```python
from build123d import *

# Parameters (mm, degrees)
SKETCH1_R           = 1
BOSS_EXTRUDE1_DEPTH = 3
FILLET_2_R          = 70


with BuildPart() as part:
    # Sketch1 → Boss-Extrude1 (new body)
    with BuildSketch(Plane.XY):
        with BuildLine():
            Line((-59.269719731, 24.533720681), (-59.269719731, 18.533720681))
            Line((-59.269719731, 18.533720681), (-45.247809755, 18.533720681))
            Line((-45.247809755, 18.533720681), (-45.247809755, -4.966279319))
            Line((-45.247809755, -4.966279319), (-59.247809755, -4.966279319))
            Line((-59.247809755, -4.966279319), (-59.247809755, -9.307077777))
            Line((-59.247809755, -9.307077777), (-51.83788451, -34.085396001))
            Line((-51.83788451, -34.085396001), (-51.83788451, -65.202303041))
            ThreePointArc((-51.83788451, -65.202303041), (-50.943230184, -66.196738704), (-49.860079932, -65.411822033))
            Line((-49.860079932, -65.411822033), (-37.838240661, -9.307077777))
            Line((-37.838240661, -9.307077777), (-37.838240661, 24.533720681))
            ThreePointArc((-37.838240661, 24.533720681), (-48.553980196, 35.249460216), (-59.269719731, 24.533720681))
        make_face()
        with Locations((-52.247809755, 20.533720681)):
            Circle(SKETCH1_R, mode=Mode.SUBTRACT)
        with Locations((-52.247809755, -6.966279319)):
            Circle(SKETCH1_R, mode=Mode.SUBTRACT)
        with BuildLine():
            Line((-45.247809755, 24.533720681), (-56.258764743, 24.533720681))
            ThreePointArc((-56.258764743, 24.533720681), (-50.753287249, 30.039198175), (-45.247809755, 24.533720681))
        make_face(mode=Mode.SUBTRACT)
    extrude(amount=BOSS_EXTRUDE1_DEPTH)

    # Скругление2
    # the kernel refuses this fillet: 70 mm, written as the material it adds along each edge
    with BuildSketch(Plane(origin=(-51.83788451, -34.085396001, 0), x_dir=(-0.28651166180092774, 0.9580767545724459, 0), z_dir=(0, 0, 1))) as fillet_2_piece_1:
        with BuildLine():
            CenterArc((FILLET_2_R * 0.146322998387, FILLET_2_R), FILLET_2_R, 253.350770917, 16.649229083)
            Line((-FILLET_2_R * 0.140188663414, FILLET_2_R * 0.0419232454276), (0, 0))
            Line((0, 0), (FILLET_2_R * 0.146322998387, 0))
        make_face()
    extrude(amount=3)
    # the kernel refuses this fillet: 70 mm, written as the material it takes off along each edge
    with BuildSketch(Plane(origin=(-59.247809755, -9.307077777, -22.444406255), x_dir=(0, 1, 0), z_dir=(0, 0, 1))) as fillet_2_2_piece_1:
        with BuildLine():
            CenterArc((11.454430765, -69.637606474), FILLET_2_R, 95.832656056, 10.816573027)
            Line((-8.601385561, -2.572233654), (0, 0))
            Line((0, 0), (4.340798458, 0))
        make_face()
    extrude(amount=47.88881251, mode=Mode.SUBTRACT)
    with BuildSketch(Plane(origin=(-37.838240661, -9.307077777, -18.538648377), x_dir=(0, 1, 0), z_dir=(0, 0, 1))) as fillet_2_2_piece_2:
        with BuildLine():
            CenterArc((FILLET_2_R * 0.10593513358, FILLET_2_R), FILLET_2_R, 257.905834548, 12.094165452)
            Line((-FILLET_2_R * 0.103583858541, FILLET_2_R * 0.0221954224179), (0, 0))
            Line((0, 0), (FILLET_2_R * 0.10593513358, 0))
        make_face()
    extrude(amount=40.077296753, mode=Mode.SUBTRACT)


solid = part.part
```
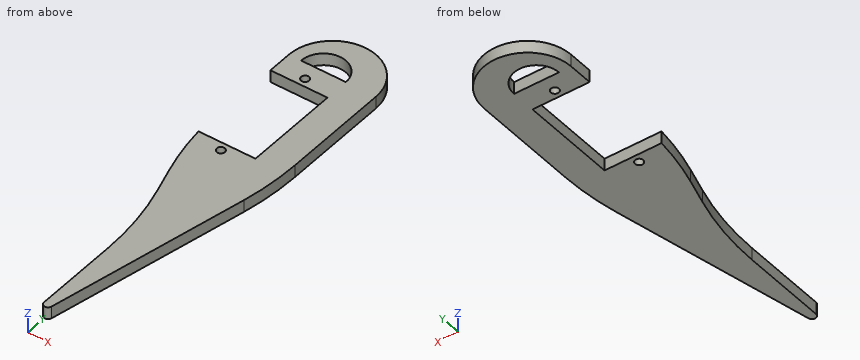
The listing builds one solid part. Answer for the finished solid, in the listing's coordinates (mm). Give positions to 0.01 mm unless a question says otherwise; leave off trailing zeros. Order: outer loops, then holes, each group sorted by start corner. A loop starts at its lowest first (then second) coordinate and runs counter-clockwise, first axis right, second up. Notation, with made-up numbers: (32.25, 58) - (76.25, 58) arc R13 cw to (76.25, 78) - close; hole circle Ø10 at (60.25, 54). An arc over 180 degrees is marked (long way). Use one line per item in the form item = value. Start each with the question number.
(1) Flat-ended cylindrical pins translate along their axes: pin 1 Ø0.9 at (y, z) = (9, 1) entering from -X; pin 2 Ø1.8 at (x, y) = (-52.25, 20.53) entering from +Z. Find the tip coordinate at first contact, or state that the pin passes through.
(2) A cutting plane is placed at C-C, the plane x = -42.5. Write down the section's boundary in (y, z).
(3) A cutting plane is placed at B-B, the plane y = 8. Write down the section's boundary in (x, z).
(4) Consider line 1 (Y direction, x = -51.75, z = 1.7); line 2 (X direction, y = 10.5, z = 1.35); line 3 (X direction, y = -26, z = 1.3). Determine where each line is inside the solid, lowest interval first. Write a range as from..to.
(5) A cutting plane is placed at A-A, the plane z = 2.5. Write down the section's boundary in (x, y), then the cut area to 3 significant figures.
Ans:
q1.pin_1 = -45.25
q1.pin_2 = through
q2.outline = (-31.06, 0) - (33.38, 0) - (33.38, 3) - (-31.06, 3) - close
q3.outline = (-45.25, 0) - (-37.84, 0) - (-37.84, 3) - (-45.25, 3) - close
q4.line_1 = -65.61..-7.83, -6.1..-4.97, 18.53..19.67, 21.4..24.53, 29.95..34.76
q4.line_2 = -45.25..-37.84
q4.line_3 = -54.28..-41.42
q5.outline = (-59.27, 18.53) - (-45.25, 18.53) - (-45.25, -4.97) - (-59.25, -4.97) arc R70 ccw to (-56.68, -17.91) - (-54.77, -24.27) arc R70 cw to (-51.84, -44.33) - (-51.84, -65.2) arc R1 ccw to (-49.86, -65.41) - (-39.39, -16.56) arc R70 ccw to (-37.84, -1.89) - (-37.84, 24.53) arc R10.72 ccw to (-59.27, 24.53) - close; hole (-56.26, 24.53) - (-45.25, 24.53) arc R5.51 ccw to start; hole circle Ø2 at (-52.25, -6.97); hole circle Ø2 at (-52.25, 20.53)
q5.area = 1,060 mm^2
